Verification items for the finished model (mm, model axes). A direction names the side the tool comes from. Round coordinates to 2 decimals unless told otherwise and drop trailing zeros. Write each loop counter-clockwise with the first axis right and the second up, starting at its lowest first coordinate (ties: lowest second). Pieces come first, ordered by that corner, then holes. Notation, with made-up numbers: (48, -19.5) - (102, -19.5) arc R22 cw to (102, 10.5) - close; hole circle Ø1 at (48.5, 49). An arc over 180 degrees is marked (long way). Write each question's results on one line, items separated by ' | '.
```python
from build123d import *

# Parameters (mm, degrees)
SKETCH1_W      = 11.9
SKETCH1_H      = 14.4
EXTRUDE1_DEPTH = 3.7
EXTRUDE2_DEPTH = 3
SKETCH4_W      = 5.6
SKETCH4_H      = 12.8
EXTRUDE3_DEPTH = 4.5


with BuildPart() as part:
    # Sketch1 → Extrude1 (new body, symmetric)
    with BuildSketch(Plane.XY):
        Rectangle(SKETCH1_W, SKETCH1_H)
    extrude(amount=EXTRUDE1_DEPTH, both=True)

    # Sketch2 → Revolve1 (revolve)
    with BuildSketch(Plane.XY):
        Polygon((5.95, 0), (5.95, 2.875), (6.425, 2.4), (20.555874546, 2.4), (22.45, 2.7), (23.95, 2.7), (23.95, 1.74), (33.95, 1.74), (33.95, 0), align=None)
    revolve(axis=Axis((0, 0, 0), (1, 0, 0)))

    # Sketch3 → Extrude2 (add, symmetric)
    with BuildSketch(Plane(origin=(0, 0, 0), x_dir=(1, 0, 0), z_dir=(0, 1, 0))):
        Polygon((-1.75, -3.7), (-1.31, -3.9), (-1.06, -3.9), (-0.85, -3.7), align=None)
        Polygon((-0.55, -3.7), (0.35, -3.7), (0.14, -3.9), (-0.11, -3.9), align=None)
        Polygon((0.65, -3.7), (1.55, -3.7), (1.34, -3.9), (1.09, -3.9), align=None)
        Polygon((1.85, -3.7), (2.75, -3.7), (2.54, -3.9), (2.29, -3.9), align=None)
    extrude(amount=EXTRUDE2_DEPTH, both=True)

    # Sketch4 → Extrude3 (cut)
    with BuildSketch(Plane.ZY.offset(5.95)):
        Rectangle(SKETCH4_W, SKETCH4_H)
    extrude(amount=-EXTRUDE3_DEPTH, mode=Mode.SUBTRACT)


solid = part.part
```
(1) Mould release check, pull along X, two halves, no side actions. Record for faces 5 (the flat face through (-4, 0, 2.8)), 6 (the flat face through (23.95, 0, -2)), 7 (the cylindrical face through (13.589, 1.29, 2.024)): released by +X, released by -X, zero draft, split by the parting line, or undercut.
Answer:
face 5: zero draft | face 6: released by +X | face 7: undercut
(2) Thickness scan on L1, parallel to X at y = 2.5, z = 3; L2, parallel to X at y = 2, z = -1; L3, parallel to Z at x = -3, y = -5.75. Record the ranges inside material, lowest first.
Answer:
L1: -5.95 to 5.95 | L2: -1.45 to 23.95 | L3: -3.7 to -2.8, 2.8 to 3.7
(3) Section check D-D (x = 26). Record the cut outline in (y, z).
Answer:
outline: circle Ø3.48 at (0, 0)
(4) Section check B-B (x = 17.5). Record the cut outline in (y, z).
Answer:
outline: circle Ø4.8 at (0, 0)
(5) Set-up check for faces 1 (the flat face through (-1.45, 0, 0)), 2 (the cylindrical face through (23.21, -0.585, -2.636)), 3 (the flat face through (33.95, 0, 0)), 4 (the conical face through (21.095, -0.539, -2.426)): record each of +Z, -Z, +X, -X, +Y, -Y from which the full face is reachable in a straight line by a thin tool's end or side.
Answer:
face 1: -X | face 2: +X | face 3: +Z, -Z, +X, +Y, -Y | face 4: none
(6) Go/stop test with flat-tipped pins: pin 1 Ø3.5 at (x, y) = (-4.5, 2.5) entering from +Z; pin 2 Ø3.5 at (x, y) = (3, -3.5) entering from +Z; pin 3 Ø4 at (x, y) = (18.5, -2.5) entering from -Z; pin 4 Ø1 at (y, z) = (1, -0.5) entering from -X. Record where each tip stops, or that it passes through.
Answer:
pin 1: z = 3.7 | pin 2: z = 3.9 | pin 3: z = -2.35 | pin 4: x = -1.45
(7) Section check A-A (z = 0). Record the cut outline in (x, y) (3 decimals), plus the area to 3 significant figures.
Answer:
outline: (-5.95, -7.2) - (5.95, -7.2) - (5.95, -2.875) - (6.425, -2.4) - (20.556, -2.4) - (22.45, -2.7) - (23.95, -2.7) - (23.95, -1.74) - (33.95, -1.74) - (33.95, 1.74) - (23.95, 1.74) - (23.95, 2.7) - (22.45, 2.7) - (20.556, 2.4) - (6.425, 2.4) - (5.95, 2.875) - (5.95, 7.2) - (-5.95, 7.2) - (-5.95, 6.4) - (-1.45, 6.4) - (-1.45, -6.4) - (-5.95, -6.4) - close | area: 237 mm2
(8) Section check C-C (x = 4). Record the cut outline in (y, z), plus the area to 3 significant figures.
Answer:
outline: (-7.2, -3.7) - (7.2, -3.7) - (7.2, 3.7) - (-7.2, 3.7) - close | area: 107 mm2
